Model file for the job. Use its own axes, mm. Coordinates: 2 decimals unless noted, no trailing zeros. Write each loop counter-clockwise with the first axis right and the second up, starting at its lowest first coordinate (ties: lowest second). Pieces come first, ordered by that corner, then holes.
Q1. Drill centre lines: probe 1 along Y at (x, z) = (12.7, 0.8); probe 2 along Y at (x, z) = (-184, 0.4); probe 3 along X at (y, z) = (388, 0.3). Where is each one in solid material? Low to high.
Q2. Band-saw the part on C-C, the plane x = -122. Write the cut outline in (y, z), plus the area to 3 significant figures.
Q3. Band-saw the part on A-A, the plane x = -209.55. Write the cut outline in (y, z), plus the area to 3 significant figures.
Q4. Band-saw the part on D-D, the plane x = 45.5. Write the cut outline in (y, z).
Q5. Pin check, flat tips, straight feed: P1, Ø2, axis at x = -50, y = 230, coming from the -Z side; P2, Ø0.5, axis at x = 171.5, z = 1, coming from the -Y side. Stop position of each tip, or through.
Q6. Band-saw the part on B-B, the plane z = 0.95. Write the cut outline in (x, y) (3 decimals), plus the area to 3 significant figures.
Autodesk Inventor part; units mm, degrees
ref_plane "YZ Plane" through (0, 0, 0) normal (1, 0, 0) x (0, 1, 0)
ref_plane "XZ Plane" through (0, 0, 0) normal (0, 1, 0) x (-1, 0, 0)
ref_plane "XY Plane" through (0, 0, 0) normal (0, 0, 1) x (1, 0, 0)
sketch "Sketch1" plane through (0, 0, 0) normal (0, 0, 1) x (1, 0, 0)
  line L0 (0, 0) -> (25.4, 0)
  line L1 (25.4, 0) -> (114.3, 127)
  line L2 (12.7, 0) -> (12.7, 419.1) construction
  line L3 (114.3, 127) -> (266.7, 127)
  line L4 (266.7, 127) -> (266.7, 419.1)
  line L5 (266.7, 419.1) -> (12.7, 419.1)
  circle A0 centre (12.7, 12.7) radius 2.0828
  circle A1 centre (12.7, 38.1) radius 2.0828
  circle A2 centre (12.7, 63.5) radius 2.0828
  circle A3 centre (12.7, 88.9) radius 2.0828
  line L6 (0, 0) -> (-88.9, 127)
  line L7 (-88.9, 127) -> (-241.3, 127)
  line L8 (-241.3, 127) -> (-241.3, 419.1)
  line L9 (-241.3, 419.1) -> (12.7, 419.1)
  dimension "d0" = 25.4
  dimension "d2" = 254
  dimension "d3" = 419.1
  dimension "d4" = 127
  dimension "d5" = 152.4
  dimension "d6" = 4.1656
  dimension "d7" = 12.7
  dimension "d10" = 25.4
extrude "Extrusion1" add sketch "Sketch1" along normal blind 1.5875
fillet "Fillet1" radius 12.7 8 edges at (25.4, 0, 0.7937) (114.3, 127, 0.7937) (266.7, 127, 0.7937) (266.7, 419.1, 0.7937) (-241.3, 419.1, 0.7937) (-241.3, 127, 0.7937) (-88.9, 127, 0.7937) (0, 0, 0.7937)
sketch "Sketch2" plane through (0, 0, 1.5875) normal (0, 0, 1) x (1, 0, 0)
  line L0 (254, 419.1) -> (-228.6, 419.1)
  line L1 (-241.3, 406.4) -> (-241.3, 139.7)
  circle A0 centre (-209.55, 384.175) radius 15.875
  circle A1 centre (-165.1, 384.175) radius 15.875
  circle A2 centre (-120.65, 384.175) radius 15.875
  circle A3 centre (-76.2, 384.175) radius 15.875
  circle A4 centre (-31.75, 384.175) radius 15.875
  circle A5 centre (12.7, 384.175) radius 15.875
  circle A6 centre (57.15, 384.175) radius 15.875
  circle A7 centre (101.6, 384.175) radius 15.875
  circle A8 centre (146.05, 384.175) radius 15.875
  circle A9 centre (190.5, 384.175) radius 15.875
  circle A10 centre (234.95, 384.175) radius 15.875
  circle A11 centre (-209.55, 339.725) radius 15.875
  circle A12 centre (-165.1, 339.725) radius 15.875
  circle A13 centre (-120.65, 339.725) radius 15.875
  circle A14 centre (-76.2, 339.725) radius 15.875
  circle A15 centre (-31.75, 339.725) radius 15.875
  circle A16 centre (12.7, 339.725) radius 15.875
  circle A17 centre (57.15, 339.725) radius 15.875
  circle A18 centre (101.6, 339.725) radius 15.875
  circle A19 centre (146.05, 339.725) radius 15.875
  circle A20 centre (190.5, 339.725) radius 15.875
  circle A21 centre (234.95, 339.725) radius 15.875
  circle A22 centre (-209.55, 295.275) radius 15.875
  circle A23 centre (-165.1, 295.275) radius 15.875
  circle A24 centre (-120.65, 295.275) radius 15.875
  circle A25 centre (-76.2, 295.275) radius 15.875
  circle A26 centre (-31.75, 295.275) radius 15.875
  circle A27 centre (12.7, 295.275) radius 15.875
  circle A28 centre (57.15, 295.275) radius 15.875
  circle A29 centre (101.6, 295.275) radius 15.875
  circle A30 centre (146.05, 295.275) radius 15.875
  circle A31 centre (190.5, 295.275) radius 15.875
  circle A32 centre (234.95, 295.275) radius 15.875
  circle A33 centre (-209.55, 250.825) radius 15.875
  circle A34 centre (-165.1, 250.825) radius 15.875
  circle A35 centre (-120.65, 250.825) radius 15.875
  circle A36 centre (-76.2, 250.825) radius 15.875
  circle A37 centre (-31.75, 250.825) radius 15.875
  circle A38 centre (12.7, 250.825) radius 15.875
  circle A39 centre (57.15, 250.825) radius 15.875
  circle A40 centre (101.6, 250.825) radius 15.875
  circle A41 centre (146.05, 250.825) radius 15.875
  circle A42 centre (190.5, 250.825) radius 15.875
  circle A43 centre (234.95, 250.825) radius 15.875
  circle A44 centre (-209.55, 206.375) radius 15.875
  circle A45 centre (-165.1, 206.375) radius 15.875
  circle A46 centre (-120.65, 206.375) radius 15.875
  circle A47 centre (-76.2, 206.375) radius 15.875
  circle A48 centre (-31.75, 206.375) radius 15.875
  circle A49 centre (12.7, 206.375) radius 15.875
  circle A50 centre (57.15, 206.375) radius 15.875
  circle A51 centre (101.6, 206.375) radius 15.875
  circle A52 centre (146.05, 206.375) radius 15.875
  circle A53 centre (190.5, 206.375) radius 15.875
  circle A54 centre (234.95, 206.375) radius 15.875
  circle A55 centre (-209.55, 161.925) radius 15.875
  circle A56 centre (-165.1, 161.925) radius 15.875
  circle A57 centre (-120.65, 161.925) radius 15.875
  circle A58 centre (-76.2, 161.925) radius 15.875
  circle A59 centre (-31.75, 161.925) radius 15.875
  circle A60 centre (12.7, 161.925) radius 15.875
  circle A61 centre (57.15, 161.925) radius 15.875
  circle A62 centre (101.6, 161.925) radius 15.875
  circle A63 centre (146.05, 161.925) radius 15.875
  circle A64 centre (190.5, 161.925) radius 15.875
  circle A65 centre (234.95, 161.925) radius 15.875
  circle A66 centre (-209.55, 117.475) radius 15.875
  circle A67 centre (-165.1, 117.475) radius 15.875
  circle A68 centre (-120.65, 117.475) radius 15.875
  circle A69 centre (-76.2, 117.475) radius 15.875
  circle A70 centre (-31.75, 117.475) radius 15.875
  circle A71 centre (12.7, 117.475) radius 15.875
  circle A72 centre (57.15, 117.475) radius 15.875
  circle A73 centre (101.6, 117.475) radius 15.875
  circle A74 centre (146.05, 117.475) radius 15.875
  circle A75 centre (190.5, 117.475) radius 15.875
  circle A76 centre (234.95, 117.475) radius 15.875
  circle A77 centre (-209.55, 73.025) radius 15.875
  circle A78 centre (-165.1, 73.025) radius 15.875
  circle A79 centre (-120.65, 73.025) radius 15.875
  circle A80 centre (-76.2, 73.025) radius 15.875
  circle A81 centre (-31.75, 73.025) radius 15.875
  circle A82 centre (12.7, 73.025) radius 15.875
  circle A83 centre (57.15, 73.025) radius 15.875
  circle A84 centre (101.6, 73.025) radius 15.875
  circle A85 centre (146.05, 73.025) radius 15.875
  circle A86 centre (190.5, 73.025) radius 15.875
  circle A87 centre (234.95, 73.025) radius 15.875
  point P0 (0, 0)
  dimension "d18" = 31.75
  dimension "d19" = 34.925
  dimension "d20" = 31.75
  dimension "d23" = 44.45
  dimension "d26" = 44.45
extrude "Extrusion2" cut sketch "Sketch2" against normal blind 1.5875 contours A0
properties part number "Funnel 2" material "Polycarbonate, Clear"
Answer sheet:
1. probe 1: y = 0 to 10.62, 14.78 to 36.02, 40.18 to 61.42, 65.58 to 86.82, 90.98 to 419.1
1. probe 2: y = 127 to 419.1
1. probe 3: x = -241.3 to -224.96, -194.14 to 266.7
2. outline: (127, 0) - (419.1, 0) - (419.1, 1.59) - (127, 1.59) - close
2. area: 464 mm2
3. outline: (127, 0) - (368.3, 0) - (368.3, 1.59) - (127, 1.59) - close; (400.05, 0) - (419.1, 0) - (419.1, 1.59) - (400.05, 1.59) - close
3. area: 413 mm2
4. outline: (28.71, 0) - (419.1, 0) - (419.1, 1.59) - (28.71, 1.59) - close
5. P1: stops at z = 0
5. P2: stops at y = 127
6. outline: (-241.3, 139.7) arc R12.7 ccw to (-228.6, 127) - (-95.512, 127) arc R12.7 cw to (-85.108, 121.583) - (-3.792, 5.417) arc R12.7 ccw to (6.612, 0) - (18.788, 0) arc R12.7 ccw to (29.192, 5.417) - (110.508, 121.583) arc R12.7 cw to (120.912, 127) - (254, 127) arc R12.7 ccw to (266.7, 139.7) - (266.7, 406.4) arc R12.7 ccw to (254, 419.1) - (-228.6, 419.1) arc R12.7 ccw to (-241.3, 406.4) - close; hole circle Ø31.75 at (-209.55, 384.175); hole circle Ø4.166 at (12.7, 12.7); hole circle Ø4.166 at (12.7, 38.1); hole circle Ø4.166 at (12.7, 63.5); hole circle Ø4.166 at (12.7, 88.9)
6. area: 162,000 mm2
